Autodesk Inventor part; units mm, degrees
ref_plane "YZ Plane" through (0, 0, 0) normal (1, 0, 0) x (0, 1, 0)
ref_plane "XZ Plane" through (0, 0, 0) normal (0, 1, 0) x (-1, 0, 0)
ref_plane "XY Plane" through (0, 0, 0) normal (0, 0, 1) x (1, 0, 0)
sketch "Sketch1" plane through (0, 0, 0) normal (1, 0, 0) x (0, 1, 0)
  line L0 (0, 0) -> (0, -33.1818)
  line L1 (8, 2.1062) -> (20, 2.1062)
  line L2 (20, 2.1062) -> (20, 0.1062)
  line L3 (20, 0.1062) -> (8, 0.1062)
  line L4 (8, 0.1062) -> (8, 2.1062)
  dimension "d3" = 2
  dimension "d4" = 40
  dimension "d28" = 16
revolve "Revolution1" add sketch "Sketch1" angle 360 about axis through (0, 0, 0) along (0, 0, -1)
sketch "Sketch2" plane through (0, 0, 2.1062) normal (0, 0, 1) x (1, 0, 0)
  point P0 (0, 0)
  point P1 (0, 16)
  dimension "d6" = 16
hole "Hole1" at (0, 16, 2.1062) direction (0, 0, -1) diameter 5 end through all
pattern_circular "Circular Pattern1" count 6 over 360 about axis through (0, 0, 1.1062) along (0, 0, -1) of "Hole1"
properties part number "PTFESeal" material "Polyethylene, High Density"
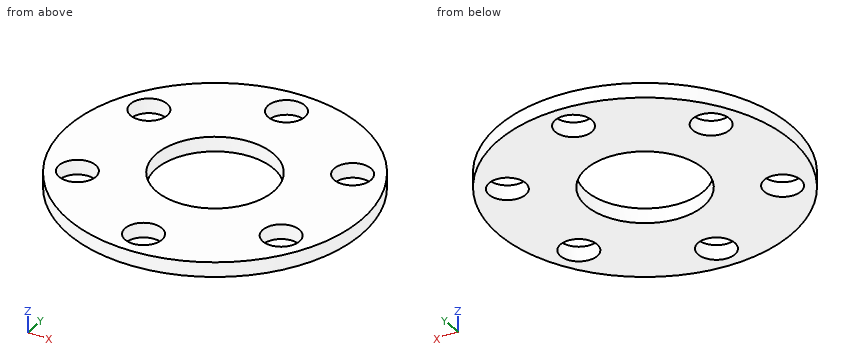
Check sheet for the modelled part. Datum: model origin and axes. Units: mm. Round coordinates to 2 decimals unless told otherwise and drop trailing zeros. Loops run counter-clockwise (first coordinate to the right, second up) from the corner with the lowest first, then second, coordinate; pieces in that order, holes last. Notation, with made-up numbers: (58, 61.25) - (95, 61.25) arc R12 cw to (95, 70.25) - close; hole circle Ø5 at (-16.75, 75). An arc over 180 degrees is marked (long way). Answer as a JSON object with one key per item and string values. Group by question number.
Q1. Sectioned sample at D-D, the plane y = 7.5. Enter the section's corners in (x, z), plus the area to 3 significant figures.
Q2. Sectioned sample at B-B, the plane y = 16. Enter the section's corners in (x, z), plus the area to 3 significant figures.
Q3. Scan lines: line 1 along X through (y, z) = (0, 1.3); line 2 along Y through (x, z) = (13.5, 0.8); line 3 along Y through (x, z) = (15, 0.7). Record each from-to range of solid material in increasing order. Write a range as [from, to].
Q4. Sectioned sample at A-A, the plane x = 0. Enter the section's corners in (y, z), plus the area to 3 significant figures.
Q5. Sectioned sample at C-C, the plane x = 6. Enter the section's corners in (y, z).
Solution:
{
 "1": {"outline": "(-18.54, 0.11) - (-16.31, 0.11) - (-16.31, 2.11) - (-18.54, 2.11) - close; (-11.41, 0.11) - (-2.78, 0.11) - (-2.78, 2.11) - (-11.41, 2.11) - close; (2.78, 0.11) - (11.41, 0.11) - (11.41, 2.11) - (2.78, 2.11) - close; (16.31, 0.11) - (18.54, 0.11) - (18.54, 2.11) - (16.31, 2.11) - close", "area": "43.4 mm²"},
 "2": {"outline": "(-12, 0.11) - (-2.5, 0.11) - (-2.5, 2.11) - (-12, 2.11) - close; (2.5, 0.11) - (12, 0.11) - (12, 2.11) - (2.5, 2.11) - close", "area": "38.0 mm²"},
 "3": {"line 1": "x = [-20, -8], [8, 20]", "line 2": "y = [-14.76, -10.47], [-5.53, 5.53], [10.47, 14.76]", "line 3": "y = [-13.23, -10.22], [-5.78, 5.78], [10.22, 13.23]"},
 "4": {"outline": "(-20, 0.11) - (-18.5, 0.11) - (-18.5, 2.11) - (-20, 2.11) - close; (-13.5, 0.11) - (-8, 0.11) - (-8, 2.11) - (-13.5, 2.11) - close; (8, 0.11) - (13.5, 0.11) - (13.5, 2.11) - (8, 2.11) - close; (18.5, 0.11) - (20, 0.11) - (20, 2.11) - (18.5, 2.11) - close", "area": "28.0 mm²"},
 "5": {"outline": "(-19.08, 0.11) - (-5.29, 0.11) - (-5.29, 2.11) - (-19.08, 2.11) - close; (5.29, 0.11) - (19.08, 0.11) - (19.08, 2.11) - (5.29, 2.11) - close"}
}
